Can you work these out from the model? Positions are in its coordinate system, mm. Face numbers are marked on the shaded views. A direction names the side the tool comes from. Round coordinates to 2 decimals unless told otherwise and drop trailing zeros. Loops run counter-clockwise (first coordinate to the right, second up) from the corner with the lowest first, then second, coordinate; pieces in that order, holes last. Notation, with made-up numbers: (40, 81.25) - (62, 81.25) arc R19 cw to (62, 99.25) - close; hole circle Ø3 at (34.5, 47.5). An arc over 180 degrees is marked (long way). Answer as CSV lines item,"result".
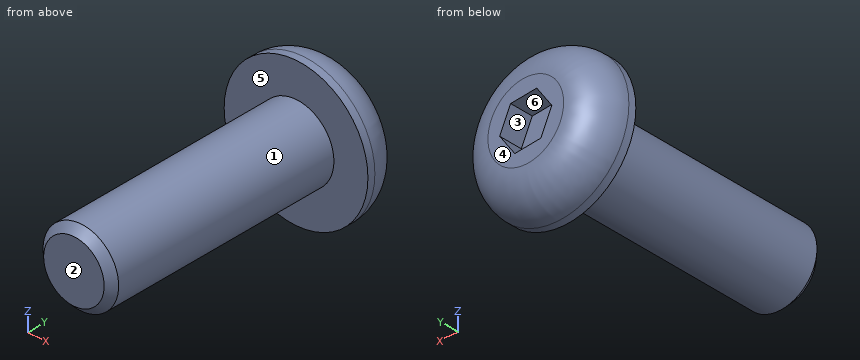
Autodesk Inventor part; units mm, degrees
ref_plane "YZ Plane" through (0, 0, 0) normal (1, 0, 0) x (0, 1, 0)
ref_plane "XZ Plane" through (0, 0, 0) normal (0, 1, 0) x (-1, 0, 0)
ref_plane "XY Plane" through (0, 0, 0) normal (0, 0, 1) x (1, 0, 0)
sketch "Boceto1" plane through (0, 0, 0) normal (0, 1, 0) x (-1, 0, 0)
  circle A0 centre (0, 0) radius 2.5
  circle A1 centre (0, 0) radius 4.75
  dimension "d0" = 5
  dimension "d1" = 9.5
extrude "Extrusión1" add sketch "Boceto1" along normal blind 2.75 contours A0 | A1
extrude "Extrusión2" add sketch "Boceto1" against normal blind 16 contours A0
thread "Rosca1"
fillet "Empalme1" radius 2.25 1 edges at (4.75, 2.75, 0)
sketch "Boceto2" plane through (0, 2.75, 0) normal (0, 1, 0) x (1, 0, 0)
  line L0 (0.7249, 1.5731) -> (1.7248, 0.1588)
  line L1 (1.7248, 0.1588) -> (0.9999, -1.4143)
  line L2 (0.9999, -1.4143) -> (-0.7249, -1.5731)
  line L3 (-0.7249, -1.5731) -> (-1.7248, -0.1588)
  line L4 (-1.7248, -0.1588) -> (-0.9999, 1.4143)
  line L5 (-0.9999, 1.4143) -> (0.7249, 1.5731)
  point P0 (0, 0)
  point P1 (0, 0)
  dimension "d9" = 3
extrude "Extrusión3" cut sketch "Boceto2" against normal blind 1.56
chamfer "Chaflán1" distance 0.5 angle 45 1 edges at (2.5, -16, 0)
properties part number "Tornillo allen cabeza boton M5x16mm"
Q1. On a 3-axis mill with a long thin cutter (end or side, diameter ignored), from which of +Z, -Z, +X, -X, +Y, -Y can I reach the whole of each face in a straight line? I mean the marked faces 4, 5 and 6. Say none if no direction works.
Checks:
face 4,"+Z, -Z, +X, -X, +Y"
face 5,"-Y"
face 6,"+Y"
Q2. Imagine slicing it at A-A (x = 0). Write out the boundary of the cut face in (y, z).
Checks:
outline,"(-16, -2) - (-15.5, -2.5) - (0, -2.5) - (0, -4.75) - (0.5, -4.75) arc R2.25 ccw to (2.75, -2.5) - (2.75, -1.51) - (1.19, -1.51) - (1.19, 1.51) - (2.75, 1.51) - (2.75, 2.5) arc R2.25 ccw to (0.5, 4.75) - (0, 4.75) - (0, 2.5) - (-15.5, 2.5) - (-16, 2) - close"
Q3. I'm going to push flat-ended pins straight in: pin 1 Ø3.5 at (x, z) = (0.5, 0) entering from +Y; pin 2 Ø1 at (y, z) = (-11.5, 2) entering from +X; pin 3 Ø5 at (y, z) = (-6, 1) entering from -X; pin 4 Ø3 at (x, y) = (-1, -10.5) entering from +Z. Where does each tip first touch, or does it pass through?
Checks:
pin 1,"y = 2.75"
pin 2,"x = 2"
pin 3,"x = -2.5"
pin 4,"z = 2.5"
Q4. Imagine slicing it at B-B (y = -10.75). Write out the boundary of the cut face in (x, z), then the cut area to 3 significant figures.
Checks:
outline,"circle Ø5 at (0, 0)"
area,"19.6 mm²"
Q5. We'd pull the mould along X, two halves only. Please class the marked faces 1, 2 and 3: pulls with the +X half, pulls with the -X half, needs draft (parallel to the pull), parting line crosses it, or undercut.
Checks:
face 1,"parting line crosses it"
face 2,"needs draft"
face 3,"undercut"
Q6. If I drill on line 1 along Y through (x, z) = (-0.5, 3.5); line 2 along X through (y, z) = (1.5, 1); line 3 along Z through (x, y) = (0, -13), over which ranges is the centre line in solid material (lowest first)? Write a range as [from, to].
Checks:
line 1,"[0, 2.5]"
line 2,"[-4.4, -1.13], [1.19, 4.4]"
line 3,"[-2.5, 2.5]"
